```python
from build123d import *

# Parameters (mm, degrees)
SKETCH1_W               = 20.32
SKETCH1_H               = 25.4
BOSS_EXTRUDE1_DEPTH     = 5.08
ELECTRONICS_HOLES_REACH = 7.08
SKETCH2_R               = 1.499997
SKETCH3_W               = 20.32
SKETCH3_H               = 10.16
BOSS_EXTRUDE2_DEPTH     = 2.54
SKETCH4_W               = 20.32
SKETCH4_H               = 22.86
CUT_EXTRUDE2_DEPTH      = 1.27
SKETCH5_R               = 1.778
PLACEMENT_HOLES_DEPTH   = 2.54
SKETCH6_W               = 15.24
SKETCH6_H               = 5.08
CUT_EXTRUDE4_DEPTH      = 9.89
BOSS_EXTRUDE3_DEPTH     = 2.54


with BuildPart() as part:
    # Sketch1 → Boss-Extrude1 (new body)
    with BuildSketch(Plane.XY):
        with Locations((10.16, 12.7)):
            Rectangle(SKETCH1_W, SKETCH1_H)
    extrude(amount=BOSS_EXTRUDE1_DEPTH)

    # Sketch2 → Electronics Holes (cut, up to next)
    with BuildSketch(Plane.XY.offset(5.08), mode=Mode.PRIVATE) as electronics_holes_sk1:
        with Locations((2.54, 22.86)):
            Circle(SKETCH2_R)
    electronics_holes_tool1 = extrude(electronics_holes_sk1.sketch, amount=-ELECTRONICS_HOLES_REACH, mode=Mode.PRIVATE) & part.part
    add(electronics_holes_tool1.solids().sort_by_distance((2.54, 22.86, 5.08))[0], mode=Mode.SUBTRACT)
    # Sketch2 → Electronics Holes (cut, up to next)
    with BuildSketch(Plane.XY.offset(5.08), mode=Mode.PRIVATE) as electronics_holes_sk2:
        with Locations((17.78, 22.86)):
            Circle(SKETCH2_R)
    electronics_holes_tool2 = extrude(electronics_holes_sk2.sketch, amount=-ELECTRONICS_HOLES_REACH, mode=Mode.PRIVATE) & part.part
    add(electronics_holes_tool2.solids().sort_by_distance((17.78, 22.86, 5.08))[0], mode=Mode.SUBTRACT)

    # Sketch3 → Boss-Extrude2 (add)
    with BuildSketch(Plane.XZ):
        with Locations((10.16, 0)):
            Rectangle(SKETCH3_W, SKETCH3_H)
    extrude(amount=-BOSS_EXTRUDE2_DEPTH)

    # Sketch4 → Cut-Extrude2 (cut)
    with BuildSketch(Plane.XY.offset(5.08)):
        with Locations((10.16, 13.97)):
            Rectangle(SKETCH4_W, SKETCH4_H)
    extrude(amount=-CUT_EXTRUDE2_DEPTH, mode=Mode.SUBTRACT)

    # Sketch5 → Placement Holes (cut)
    with BuildSketch(Plane(origin=(0, 2.54, 0), x_dir=(1, 0, 0), z_dir=(0, 1, 0))):
        with Locations((17.78, 2.54)):
            Circle(SKETCH5_R)
        with Locations((2.54, 2.54)):
            Circle(SKETCH5_R)
    extrude(amount=-PLACEMENT_HOLES_DEPTH, mode=Mode.SUBTRACT)

    # Sketch6 → Cut-Extrude4 (cut, through all)
    with BuildSketch(Plane.XY.offset(3.81)):
        with Locations((10.16, 5.08)):
            Rectangle(SKETCH6_W, SKETCH6_H)
    extrude(amount=-CUT_EXTRUDE4_DEPTH, mode=Mode.SUBTRACT)

    # Sketch7 → Boss-Extrude3 (add)
    with BuildSketch(Plane.ZY.offset(-10.16)):
        Polygon((0, 25.4), (-5.08, 2.54), (3.81, 2.54), (3.81, 25.4), align=None)
    boss_extrude3 = extrude(amount=BOSS_EXTRUDE3_DEPTH)

    # Mirror1: Boss-Extrude3 across plane
    add(boss_extrude3.mirror(Plane.ZY.offset(-10.16)))


solid = part.part
```
Design review of the part built by this model. Coordinates are the model's own, in mm. A direction names the side the tool comes from. Give positions to 0.01 mm unless a question says otherwise; leave off trailing zeros. Loops run counter-clockwise (first coordinate to the right, second up) from the corner with the lowest first, then second, coordinate; pieces in that order, holes last. Notation, with made-up numbers: (21.5, 35) -> (74.5, 35) arc R11 cw to (74.5, 48) -> close; hole circle Ø5 at (69, 12). An arc over 180 degrees is marked (long way). One line per item, written item: value.
Q1. We need section B-B on z = -2.54. Give the boundary of the cut face in (x, y), and give its area (3 significant figures).
Numbers:
outline: (0, 0) -> (0.76, 0) -> (0.76, 2.54) -> (0, 2.54) -> close; (4.32, 0) -> (16, 0) -> (16, 2.54) -> (12.7, 2.54) -> (12.7, 13.97) -> (7.62, 13.97) -> (7.62, 2.54) -> (4.32, 2.54) -> close; (19.56, 0) -> (20.32, 0) -> (20.32, 2.54) -> (19.56, 2.54) -> close
area: 91.6 mm^2
Q2. For pin 1 Ø4 at (x, y) = (17.5, 9.5) entering from -Z; pin 2 Ø4 at (x, y) = (14, 15) entering from -Z; pin 3 Ø2 at (x, z) = (17.78, -2.54) entering from +Y; pin 4 Ø4 at (x, y) = (17.78, 22.86) entering from +Z, all flat-tipped, find the tip position at first contact; note any pin that passes through.
Numbers:
pin 1: stops at z = 0
pin 2: stops at z = -2.65
pin 3: passes through
pin 4: stops at z = 3.81
Q3. Draft analysis for pull direction Y (two halves, no side actions). For faces 1 (the cylindrical face through (17.455, 21.396, 1.932)), 2 (the flat face through (10, 1, 5.08)), 3 (the flat face through (10.124, 14.13, -2.504)), state which applies: pulls with the +Y half, pulls with the -Y half, needs draft (parallel to the pull), parting line crosses it, or undercut.
Numbers:
face 1: undercut
face 2: needs draft
face 3: pulls with the +Y half
Q4. We need section C-C on x = 5.25. Give the boundary of the cut face in (y, z).
Numbers:
outline: (0, -5.08) -> (2.54, -5.08) -> (2.54, 5.08) -> (0, 5.08) -> close; (7.62, 0) -> (25.4, 0) -> (25.4, 3.81) -> (7.62, 3.81) -> close
Q5. We need section A-A on y = 4.25. Give the boundary of the cut face in (x, z).
Numbers:
outline: (0, 0) -> (2.54, 0) -> (2.54, 3.81) -> (0, 3.81) -> close; (7.62, -4.7) -> (12.7, -4.7) -> (12.7, 3.81) -> (7.62, 3.81) -> close; (17.78, 0) -> (20.32, 0) -> (20.32, 3.81) -> (17.78, 3.81) -> close
Q6. For L1, parallel to X at y = 1.35, z = -2.54; L2, parallel to X at y = 22.75, z = 2.5; L3, parallel to Z at x = 2.54, y = 1.85, list the stretches that pass through material, from the lowest coordinate up.
Numbers:
L1: x = 0 to 0.76, 4.32 to 16, 19.56 to 20.32
L2: x = 0 to 1.04, 4.04 to 16.28, 19.28 to 20.32
L3: z = -5.08 to -4.32, -0.76 to 5.08
Q7. Machinability: for faces 4 (the cylindrical face through (1.1, 1.3, -1.5)), 5 (the flat face through (7.62, 9, -1)), 6 (the flat face through (10, 14, 3.81)), 7 (the flat face through (2.54, 5, 2)), 8 (the flat face through (4, 14, 0)), which of the approach directions +Z, -Z, +X, -X, +Y, -Y give a long, thin tool a straight path to every point of the face, cutting with its end or side? Answer none if there is none.
Numbers:
face 4: +Y, -Y
face 5: -Z
face 6: +Z, +X, -X, +Y
face 7: +Z, -Z
face 8: -Z, -X, +Y
Q8. We need section D-D on x = 17. Give the boundary of the cut face in (y, z), and give its area (3 significant figures).
Numbers:
outline: (0, -5.08) -> (2.54, -5.08) -> (2.54, -4.14) -> (0, -4.14) -> close; (0, -0.94) -> (2.54, -0.94) -> (2.54, 5.08) -> (0, 5.08) -> close; (7.62, 0) -> (21.58, 0) -> (21.58, 3.81) -> (7.62, 3.81) -> close; (24.14, 0) -> (25.4, 0) -> (25.4, 3.81) -> (24.14, 3.81) -> close
area: 75.7 mm^2
